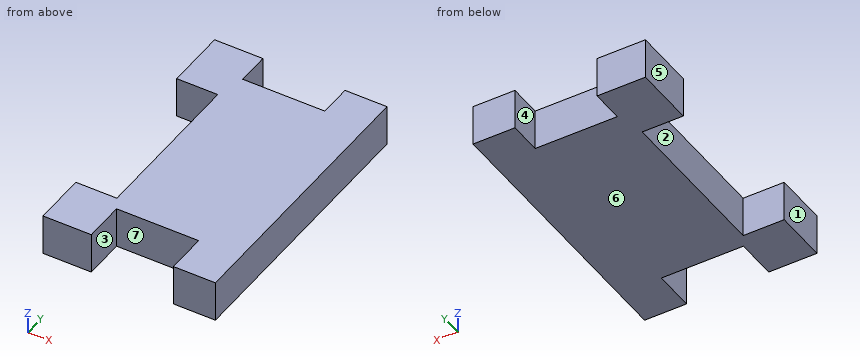
Autodesk Inventor part; units mm, degrees
ref_plane "YZ Plane" through (0, 0, 0) normal (1, 0, 0) x (0, 1, 0)
ref_plane "XZ Plane" through (0, 0, 0) normal (0, 1, 0) x (-1, 0, 0)
ref_plane "XY Plane" through (0, 0, 0) normal (0, 0, 1) x (1, 0, 0)
sketch "Sketch1" plane through (0, 0, 0) normal (0, 0, 1) x (1, 0, 0)
  line L0 (5.4369, 31.5378) -> (26.4369, 31.5378)
  line L1 (26.4369, 31.5378) -> (26.4369, -2.4622)
  line L2 (26.4369, -2.4622) -> (5.4369, -2.4622)
  line L3 (5.4369, -2.4622) -> (5.4369, 31.5378)
  dimension "d3" = 21
  dimension "d4" = 34
extrude "Extrusion1" add sketch "Sketch1" along normal blind 5
sketch "Sketch2" plane through (5.4369, -2.4622, 0) normal (0, -1, 0) x (1, 0, 0)
  line L0 (0, 5) -> (21, 5)
  line L1 (3, 5) -> (18.7735, 5)
  line L2 (3, 5) -> (5.8868, 0)
  line L3 (0, 0) -> (21, 0)
  line L4 (3, 5) -> (8.7735, 5) construction
  line L5 (18.7735, 5) -> (15.8868, 0)
  line L6 (18.7735, 5) -> (24.547, 5) construction
  line L7 (15.8868, 0) -> (5.8868, 0)
  line L8 (5.8868, 0) -> (5.8868, 5)
  line L9 (15.8868, 5) -> (15.8868, 0)
  point P0 (-5.4369, 0)
  dimension "d8" = 3
  dimension "d9" = 60
  dimension "d10" = 120
  dimension "d32" = 10
extrude "Extrusion2" cut sketch "Sketch2" against normal blind 5 contours L0 L9 L3 L8
ref_plane "Work Plane1" through (5.4369, 15.0378, 0) normal (0, 1, 0) x (1, 0, 0)
mirror "Mirror1" about plane through (5.4369, 15.0378, 0) normal (0, 1, 0) of "Extrusion2"
sketch "Sketch3" plane through (5.4369, -2.4622, 0) normal (-1, 0, 0) x (0, 0, 1)
  line L0 (0, 34) -> (5, 34)
  line L1 (0, 1) -> (0, 34)
  line L2 (0, 34) -> (5, 34)
  line L3 (5, 34) -> (5, 0)
  line L4 (5, 6.5) -> (5, 26.5)
  line L5 (5, 6.5) -> (0, 6.5)
  line L6 (5, 6.5) -> (10, 6.5) construction
  line L7 (5, 26.5) -> (0, 26.5)
  line L8 (5, 26.5) -> (10, 26.5) construction
  line L9 (0, 26.5) -> (0, 6.5)
  dimension "d24" = 20
  dimension "d25" = 6.5
  dimension "d28" = 180
  dimension "d31" = 90
extrude "Extrusion3" cut sketch "Sketch3" against normal blind 5 contours L7 L3 L5 L1
sketch "Sketch4" plane through (0, 0, 5) normal (0, 0, 1) x (1, 0, 0)
  point P0 (0, 0)
Could you check a few things on this model? Use its own coordinates, in mm. Face numbers are marked on the shaded views. A direction names the side the tool comes from. Round coordinates to 2 decimals unless told otherwise and drop trailing zeros. Order: outer loops, then holes, each group sorted by start corner. A loop starts at its lowest first (then second) coordinate and runs counter-clockwise, first axis right, second up. Notation, with made-up numbers: M 7,82.5 L 13,82.5 A25 ccw 13,94.5 Z; hole C -19.75,-34 d2. An arc over 180 degrees is marked long. One line per question, with ' | ' between items. Start each with the question number.
(1) Suppose I cut it at A-A on x = 10. List the corners of the cut face in (y, z) for me.
(2) Thinking about a two-plate mould opening in X: for the marked faces 5, 6 and 7, which applies, +X half, -X half, draft (parallel to the pull), parting line (faces both ways), or undercut?
(3) For the marked faces 1, 2, 3 and 4, which set-ups out of +Z, -Z, +X, -X, +Y, -Y let a thin tool reach every point of the face, with its end or its side?
(4) Suppose I cut it at D-D on x = 17.25. List the corners of the cut face in (y, z) for me, then the cut area to 3 significant figures.
(5) Suppose I cut it at B-B on y = 1. List the corners of the cut face in (x, z) for me, then the cut area to 3 significant figures.
(6) For P1, Ø2.5, axis at x = 15.5, z = 1.5, coming from the -Y side, with a flat end and sliding along its axis, tell me the tip position at first contact or that it passes through.
(7) Please list where these lines run through material, in increasing order: line 1 along Y through (x, z) = (9, 2.05); line 2 along X through (y, z) = (15, 4.7); line 3 along Y through (x, z) = (14, 0.7).
(8) Suppose I cut it at C-C on z = 1.7. List the corners of the cut face in (x, y) for me, then the cut area to 3 significant figures.
Geometry results:
1) outline: M -2.46,0 L 4.04,0 L 4.04,5 L -2.46,5 Z; M 24.04,0 L 31.54,0 L 31.54,5 L 24.04,5 Z
2) face 5: -X half | face 6: draft | face 7: undercut
3) face 1: +Z, -Z, -X, +Y, -Y | face 2: +Z, -Z, -X | face 3: +Z, -Z, -Y | face 4: +Z, -Z, +Y
4) outline: M 2.54,0 L 27.54,0 L 27.54,5 L 2.54,5 Z | area: 125 mm²
5) outline: M 5.44,0 L 11.32,0 L 11.32,5 L 5.44,5 Z; M 21.32,0 L 26.44,0 L 26.44,5 L 21.32,5 Z | area: 55.0 mm²
6) P1: y = 2.54
7) line 1: -2.46 to 4.04, 24.04 to 31.54 | line 2: 10.44 to 26.44 | line 3: 2.54 to 27.54
8) outline: M 5.44,-2.46 L 11.32,-2.46 L 11.32,2.54 L 21.32,2.54 L 21.32,-2.46 L 26.44,-2.46 L 26.44,31.54 L 21.32,31.54 L 21.32,27.54 L 11.32,27.54 L 11.32,31.54 L 5.44,31.54 L 5.44,24.04 L 10.44,24.04 L 10.44,4.04 L 5.44,4.04 Z | area: 524 mm²
